```python
from build123d import *

# Parameters (mm, degrees)
SKETCH074_R     = 1.5
SKETCH074_R_2   = 12.75
SKETCH074_R_3   = 6.25
PAD042_DEPTH    = 15
SKETCH060_R     = 12.75
SKETCH060_R_2   = 6.25
PAD043_DEPTH    = 25
POCKET036_DEPTH = 10.5


with BuildPart() as part:
    # Sketch074 → Pad042 (new body)
    with BuildSketch(Plane.XY):
        with BuildLine():
            ThreePointArc((-24.8, 46), (-29.219417, 44.169417), (-31.05, 39.75))
            Line((-31.05, 39.75), (-31.05, -39.75))
            ThreePointArc((-31.05, -39.75), (-29.219417, -44.169417), (-24.8, -46))
            Line((-24.8, -46), (70.8, -46))
            ThreePointArc((70.8, -46), (75.219417, -44.169417), (77.05, -39.75))
            Line((77.05, -39.75), (77.05, 39.75))
            ThreePointArc((77.05, 39.75), (75.219417, 44.169417), (70.8, 46))
            Line((70.8, 46), (-24.8, 46))
        make_face()
        with Locations((-24.8, 39.75)):
            Circle(SKETCH074_R, mode=Mode.SUBTRACT)
        with Locations((70.8, 39.75)):
            Circle(SKETCH074_R, mode=Mode.SUBTRACT)
        with Locations((-24.8, -39.75)):
            Circle(SKETCH074_R, mode=Mode.SUBTRACT)
        with Locations((70.8, -39.75)):
            Circle(SKETCH074_R, mode=Mode.SUBTRACT)
        Circle(SKETCH074_R_2, mode=Mode.SUBTRACT)
        with Locations((46, 0)):
            Circle(SKETCH074_R_2, mode=Mode.SUBTRACT)
        with Locations((23, 0)):
            Circle(SKETCH074_R_3, mode=Mode.SUBTRACT)
    extrude(amount=-PAD042_DEPTH)

    # Sketch060 → Pad043 (join)
    with BuildSketch(Plane(origin=(0, 0, 0), x_dir=(1, 0, 0), z_dir=(0, 0, -1))):
        with BuildLine():
            ThreePointArc((0, 18.75), (-18.75, 0), (0, -18.75))
            Line((0, -18.75), (46, -18.75))
            ThreePointArc((46, -18.75), (64.75, 0), (46, 18.75))
            Line((46, 18.75), (0, 18.75))
        make_face()
        Circle(SKETCH060_R, mode=Mode.SUBTRACT)
        with Locations((46, 0)):
            Circle(SKETCH060_R, mode=Mode.SUBTRACT)
        with Locations((23, 0)):
            Circle(SKETCH060_R_2, mode=Mode.SUBTRACT)
    extrude(amount=PAD043_DEPTH)

    # Sketch064 → Pocket036 (cut)
    with BuildSketch(Plane(origin=(0, 0, 0), x_dir=(1, 0, 0), z_dir=(0, 0, -1))):
        with BuildLine():
            ThreePointArc((21.445946, 17.373296), (-27.6, 0), (21.445946, -17.373296))
            ThreePointArc((24.554054, -17.373296), (23, -16.63223), (21.445946, -17.373296))
            ThreePointArc((24.554054, -17.373296), (73.6, 0), (24.554054, 17.373296))
            ThreePointArc((21.445946, 17.373296), (23, 16.63223), (24.554054, 17.373296))
        make_face()
    extrude(amount=POCKET036_DEPTH, mode=Mode.SUBTRACT)


solid = part.part
```
Could you check a few things on this model? Use its own coordinates, in mm. A direction names the side the tool comes from. Coordinates: 2 decimals unless noted, no trailing zeros. Order: outer loops, then holes, each group sorted by start corner. A loop starts at its lowest first (then second) coordinate and runs counter-clockwise, first axis right, second up. Notation, with made-up numbers: M -25.75,79 L 25.25,79 A20 cw 25.25,99 Z; hole C -14.75,-3.75 d10. An arc over 180 degrees is marked long. Use a Markdown table: item, result. Add a question column.
Q1. I want a section at D-D on z = -21. List the corners of the cut face in (x, y) for me, then the cut area to 3 significant figures.
Q2. Which directions (+Z, -Z, +X, -X, +Y, -Y) give clear straight access to the entire face, cutting with the end or side of a thin tool? Please do faces 5 (the flat face through (23, 18.75, -20)), 6 (the flat face through (22, 21, 0)), 7 (the cylindrical face through (73.584, 0.951, -5.176)), 8 (the cylindrical face through (64.745, 0.412, -19.93)), 9 (the flat face through (24, 46, -7)).
Q3. I want a section at B-B on x = 23. List the corners of the cut face in (y, z) for me, then the cut area to 3 significant figures.
Q4. I want a section at A-A on y = 0. List the corners of the cut face in (x, z) for me.
Q5. We'd pull the mould along Y, two halves only. Please class faces 1 (the cylindrical face through (-18.745, -0.412, -19.93)), 2 (the cylindrical face through (23.025, 16.632, -5.176)), 3 (the flat face through (23, -18.75, -20)), 4 (the flat face through (32, 0, -25)): pulls with the +Y half, pulls with the -Y half, needs draft (parallel to the pull), parting line crosses it, or undercut.
Q6. I'm going to push flat-ended pins straight in: pin 1 (5 mm diameter, centred on x = 70.8, y = 39.75, fed in from +Z); pin 2 (4 mm diameter, centred on x = 29, z = -20, fed in from -Y); pin 3 (3 mm diameter, centred on x = 62.5, y = -24, fed in from -Z). Where does each tip first touch, or does it pass through?
Q7. I want a section at C-C on z = -5.75. List the corners of the cut face in (x, y) for me.
Q8. If I drill on L1, parallel to X at y = 0, z = -13.75; L2, parallel to Y at x = -24.8, z = -9.75; L3, parallel to X at y = 0, z = -7.5, over which ranges is the centre line in solid material (lowest first)?
Checked values:
| question | item | result |
|---|---|---|
| 1 | outline | M 0,-18.75 L 46,-18.75 A18.75 ccw 46,18.75 L 0,18.75 A18.75 ccw Z; hole C 0,0 d25.5; hole C 23,0 d12.5; hole C 46,0 d25.5 |
| 1 | area | 1,690 mm² |
| 2 | face 5 | -Z, +X, -X, +Y |
| 2 | face 6 | +Z, +X, -X, +Y, -Y |
| 2 | face 7 | +Z |
| 2 | face 8 | -Z, +X |
| 2 | face 9 | +Z, -Z, +X, -X, +Y |
| 3 | outline | M -46,-15 L -18.75,-15 L -18.75,-25 L -6.25,-25 L -6.25,-10.5 L -16.63,-10.5 L -16.63,0 L -46,0 Z; M 6.25,-25 L 18.75,-25 L 18.75,-15 L 46,-15 L 46,0 L 16.63,0 L 16.63,-10.5 L 6.25,-10.5 Z |
| 3 | area | 1,220 mm² |
| 4 | outline | M -31.05,-15 L -18.75,-15 L -18.75,-25 L -12.75,-25 L -12.75,-10.5 L -27.6,-10.5 L -27.6,0 L -31.05,0 Z; M 12.75,-25 L 16.75,-25 L 16.75,-10.5 L 12.75,-10.5 Z; M 29.25,-25 L 33.25,-25 L 33.25,-10.5 L 29.25,-10.5 Z; M 58.75,-25 L 64.75,-25 L 64.75,-15 L 77.05,-15 L 77.05,0 L 73.6,0 L 73.6,-10.5 L 58.75,-10.5 Z |
| 5 | face 1 | parting line crosses it |
| 5 | face 2 | undercut |
| 5 | face 3 | pulls with the -Y half |
| 5 | face 4 | needs draft |
| 6 | pin 1 | z = 0 |
| 6 | pin 2 | y = -18.75 |
| 6 | pin 3 | z = -15 |
| 7 | outline | M -31.05,-39.75 A6.25 ccw -24.8,-46 L 70.8,-46 A6.25 ccw 77.05,-39.75 L 77.05,39.75 A6.25 ccw 70.8,46 L -24.8,46 A6.25 ccw -31.05,39.75 Z; hole C -24.8,-39.75 d3; hole C -24.8,39.75 d3; hole M 21.45,-17.37 A2 cw 24.55,-17.37 A27.6 ccw long 24.55,17.37 A2 cw 21.45,17.37 A27.6 ccw long Z; hole C 70.8,-39.75 d3; hole C 70.8,39.75 d3 |
| 8 | L1 | -31.05 to -12.75, 12.75 to 16.75, 29.25 to 33.25, 58.75 to 77.05 |
| 8 | L2 | -46 to -41.25, -38.25 to -12.11, 12.11 to 38.25, 41.25 to 46 |
| 8 | L3 | -31.05 to -27.6, 73.6 to 77.05 |
